The figure shows three views and two pictorial views of one solid part (mm, origin at its lowest corner). Answer the questions. A direction names the side the tool comes from. Round coordinates to 2 decimals unless told otherwise and drop trailing zeros. Loops run counter-clockwise (first coordinate to the right, second up) from the corner with the lowest first, then second, coordinate; pieces in that order, holes last. Notation, with made-up numbers: (68, 33) -> (90, 33) arc R16 cw to (90, 60) -> close; hole circle Ø5 at (4.25, 64.25). An arc over 180 degrees is marked (long way). Put each result on its own line as item: value.
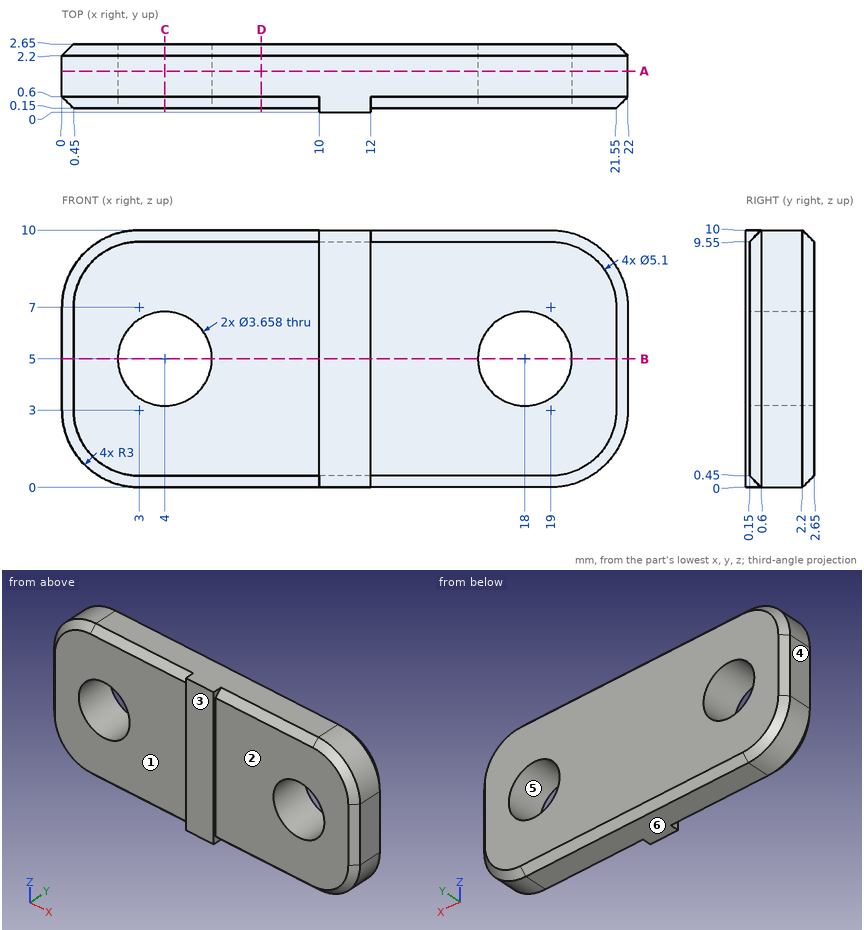
Item 1: The part is cut by section D-D (x = 7.75). Determine the outline of the cut face in (y, z).
Derived:
outline: (0.15, 0.45) -> (0.6, 0) -> (2.2, 0) -> (2.65, 0.45) -> (2.65, 9.55) -> (2.2, 10) -> (0.6, 10) -> (0.15, 9.55) -> close
Item 2: The part is cut by section B-B (z = 5). Determine the outline of the cut face in (x, y), then the cut area to 3 significant figures.
Derived:
outline: (0, 0.6) -> (0.45, 0.15) -> (2.17, 0.15) -> (2.17, 2.65) -> (0.45, 2.65) -> (0, 2.2) -> close; (5.83, 0.15) -> (10, 0.15) -> (10, 0) -> (12, 0) -> (12, 0.15) -> (16.17, 0.15) -> (16.17, 2.65) -> (5.83, 2.65) -> close; (19.83, 0.15) -> (21.55, 0.15) -> (22, 0.6) -> (22, 2.2) -> (21.55, 2.65) -> (19.83, 2.65) -> close
area: 36.6 mm^2
Item 3: Find the intervals of material crossed by line 1 along Z through (x, y) = (18, 1.85); line 2 along X through (y, z) = (1.3, 4.75); line 3 along Y through (x, z) = (2, 7), in increasing order.
Derived:
line 1: z = 0 to 3.17, 6.83 to 10
line 2: x = 0 to 2.19, 5.81 to 16.19, 19.81 to 22
line 3: y = 0.15 to 2.65
Item 4: For a pull along X with two mould halves and no side action, classify the marked faces 4, 5 and 6 as pulls with the +X half, pulls with the -X half, needs draft (parallel to the pull), parting line crosses it, or undercut.
Derived:
face 4: pulls with the -X half
face 5: undercut
face 6: needs draft
Item 5: The part is cut by section A-A (y = 1.6). Determine the outline of the cut face in (x, z).
Derived:
outline: (0, 3) arc R3 ccw to (3, 0) -> (19, 0) arc R3 ccw to (22, 3) -> (22, 7) arc R3 ccw to (19, 10) -> (3, 10) arc R3 ccw to (0, 7) -> close; hole circle Ø3.66 at (4, 5); hole circle Ø3.66 at (18, 5)
Item 6: Flat-ended cylindrical pins translate along their axes: pin 1 Ø4.5 at (x, z) = (17, 6) entering from -Y; pin 2 Ø0.7 at (y, z) = (0.5, 2.5) entering from +X (1 decimal); pin 3 Ø2 at (x, z) = (18, 5) entering from -Y. Find the tip coordinate at first contact, or state that the pin passes through.
Derived:
pin 1: stops at y = 0.15
pin 2: stops at x = 22
pin 3: passes through
Item 7: The part is cut by section C-C (x = 4). Determine the outline of the cut face in (y, z).
Derived:
outline: (0.15, 0.45) -> (0.6, 0) -> (2.2, 0) -> (2.65, 0.45) -> (2.65, 3.17) -> (0.15, 3.17) -> close; (0.15, 6.83) -> (2.65, 6.83) -> (2.65, 9.55) -> (2.2, 10) -> (0.6, 10) -> (0.15, 9.55) -> close
Item 8: Which of the six approach directions +Z, -Z, +X, -X, +Y, -Y give full straight-line access (tool end or side, diameter ignored) to the marked faces 1, 2 and 3?
Derived:
face 1: +Z, -Z, -X, -Y
face 2: +Z, -Z, +X, -Y
face 3: +Z, -Z, +X, -X, -Y
